Part model, mm, in its own coordinate system. Face numbers are marked on the shaded views. Give positions to 0.01 mm unless a question says otherwise; leave off trailing zeros. Order: outer loops, then holes, each group sorted by start corner. A loop starts at its lowest first (then second) coordinate and runs counter-clockwise, first axis right, second up. Notation, with made-up numbers: M 74.25,39.25 L 84.25,39.25 A3 cw 84.25,43.25 Z; hole C 9.5,-4.5 d11. An arc over 180 degrees is marked long. Return JSON: item names as keys, results as strings.
from build123d import *

# Parameters (mm, degrees)
F0_W     = 355.6
F0_H     = 203.2
F1_DEPTH = 254
F5_DEPTH = 50.8
F6_R     = 19.05
F7_DEPTH = 50.8
F8_R     = 19.05
F9_DEPTH = 50.8


with BuildPart() as f1:
    # F0 (on Front) → F1 (new body)
    with BuildSketch(Plane.XZ):
        with Locations((177.8, 101.6)):
            Rectangle(F0_W, F0_H)
        with Locations((-177.8, 101.6)):
            Rectangle(F0_W, F0_H)
        Polygon((355.6, 203.2), (355.6, 0), (660.4, 203.2), align=None)
        Polygon((-660.4, 203.2), (-355.6, 0), (-355.6, 203.2), align=None)
    extrude(amount=F1_DEPTH)

    # F4 (on face) + F3 (on face) → F5 (join)
    with BuildSketch(Plane.XZ.offset(254)):
        with BuildLine():
            ThreePointArc((-240.525891, 53.34), (-236.806147, 44.359744), (-227.825891, 40.64))
            Line((-227.825891, 40.64), (-202.425891, 40.64))
            ThreePointArc((-202.425891, 40.64), (-193.445635, 44.359744), (-189.725891, 53.34))
            Line((-189.725891, 53.34), (-189.725891, 129.54))
            ThreePointArc((-189.725891, 129.54), (-193.445635, 138.520256), (-202.425891, 142.24))
            Line((-202.425891, 142.24), (-227.825891, 142.24))
            ThreePointArc((-227.825891, 142.24), (-236.806147, 138.520256), (-240.525891, 129.54))
            Line((-240.525891, 129.54), (-240.525891, 53.34))
        make_face()
    with BuildSketch(Plane.XZ.offset(254)):
        with BuildLine():
            ThreePointArc((233.048756, 116.839396), (229.329012, 125.819652), (220.348756, 129.539396))
            Line((220.348756, 129.539396), (194.948756, 129.539396))
            ThreePointArc((194.948756, 129.539396), (185.9685, 125.819652), (182.248756, 116.839396))
            Line((182.248756, 116.839396), (182.248756, 53.339396))
            ThreePointArc((182.248756, 53.339396), (185.9685, 44.35914), (194.948756, 40.639396))
            Line((194.948756, 40.639396), (220.348756, 40.639396))
            ThreePointArc((220.348756, 40.639396), (229.329012, 44.35914), (233.048756, 53.339396))
            Line((233.048756, 53.339396), (233.048756, 116.839396))
        make_face()
    extrude(amount=F5_DEPTH)

    # F6 (on face) → F7 (cut)
    with BuildSketch(Plane.YZ.offset(233.048756)):
        with Locations((-279.4, 85.089396)):
            Circle(F6_R)
    extrude(amount=-F7_DEPTH, mode=Mode.SUBTRACT)

    # F8 (on face) → F9 (cut)
    with BuildSketch(Plane(origin=(-240.525891, 0, 0), x_dir=(0, -1, 0), z_dir=(-1, 0, 0))):
        with Locations((279.4, 91.44)):
            Circle(F8_R)
    extrude(amount=-F9_DEPTH, mode=Mode.SUBTRACT)


solid = f1.part
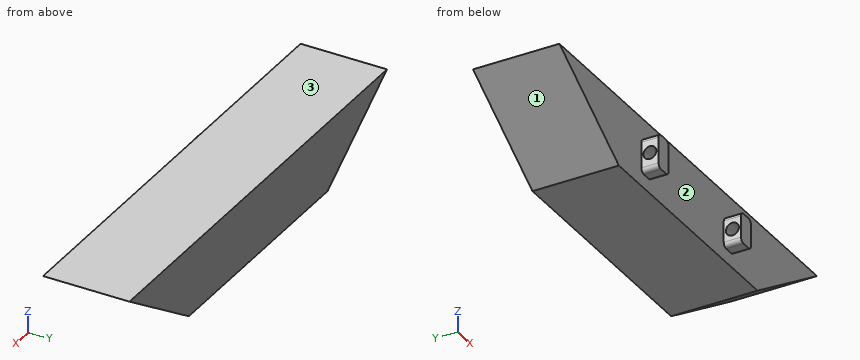
Q1. Probe line 1 along X through (y, z) = (-283.5, 114); line 2 along Z through (x, y) = (-207, -279); line 3 along Z through (x, y) = (195, -279). List the from-to ranges inside material, lowest first.
Established:
{"line 1": "x = -240.53 to -189.73, 182.25 to 233.05", "line 2": "z = 40.64 to 72.39, 110.49 to 142.24", "line 3": "z = 40.64 to 66.04, 104.14 to 129.54"}
Q2. Two-plate mould, pull along X, no slides. Class the marked faces 1, 2 and 3: +X half, -X half, draft (parallel to the pull), parting line (faces both ways), or undercut.
Established:
{"face 1": "-X half", "face 2": "undercut", "face 3": "draft"}
Q3. Band-saw the part on C-C (z = 155.5). Give the cut face in (x, y), then the cut area to 3 significant figures.
Established:
{"outline": "M -588.85,-254 L 588.85,-254 L 588.85,0 L -588.85,0 Z", "area": "299,000 mm²"}
Q4. Band-saw the part on A-A (y = -279.4). Give the cut face in (x, z), then the cut area to 3 significant figures.
Established:
{"outline": "M -240.53,53.34 A12.7 ccw -227.83,40.64 L -202.43,40.64 A12.7 ccw -189.73,53.34 L -189.73,72.39 L -240.53,72.39 Z; M -240.53,110.49 L -189.73,110.49 L -189.73,129.54 A12.7 ccw -202.43,142.24 L -227.83,142.24 A12.7 ccw -240.53,129.54 Z; M 182.25,53.34 A12.7 ccw 194.95,40.64 L 220.35,40.64 A12.7 ccw 233.05,53.34 L 233.05,66.04 L 182.25,66.04 Z; M 182.25,104.14 L 233.05,104.14 L 233.05,116.84 A12.7 ccw 220.35,129.54 L 194.95,129.54 A12.7 ccw 182.25,116.84 Z", "area": "5,530 mm²"}
Q5. Pin check, flat tips, straight feed: pin 1 (15 mm diameter, centred on y = -272, z = 99, fed in from -X); pin 2 (12.5 mm diameter, centred on x = 207, y = -269, fed in from +Z); pin 3 (15 mm diameter, centred on y = -281.5, z = 74.5, fed in from +X). Stop position of each tip, or through.
Established:
{"pin 1": "stops at x = 182.25", "pin 2": "stops at z = 129.54", "pin 3": "stops at x = -189.73"}
Q6. Band-saw the part on B-B (x = -141). Give the cut face in (y, z).
Established:
{"outline": "M -254,0 L 0,0 L 0,203.2 L -254,203.2 Z"}
